from build123d import *

# Parameters (mm, degrees)
SKETCH1_R           = 3
BOSS_EXTRUDE1_DEPTH = 3
FILLET1_R           = 1.5
SKETCH2_R           = 1.5
BOSS_EXTRUDE2_DEPTH = 12.7


with BuildPart() as part:
    # Sketch1 → Boss-Extrude1 (new body)
    with BuildSketch(Plane(origin=(0, 0, 0), x_dir=(1, 0, 0), z_dir=(0, 1, 0))):
        Circle(SKETCH1_R)
    extrude(amount=BOSS_EXTRUDE1_DEPTH)

    # Fillet1
    fillet1_edges = [part.edges().sort_by_distance(p)[0] for p in [
        (-3, 3, 0),
    ]]
    fillet(fillet1_edges, radius=FILLET1_R)

    # Sketch2 → Boss-Extrude2 (add)
    with BuildSketch(Plane.XZ):
        Circle(SKETCH2_R)
    extrude(amount=BOSS_EXTRUDE2_DEPTH)


solid = part.part
Can you work these out from the model? Positions are in its coordinate system, mm. Give positions to 0.01 mm unless a question says otherwise; leave off trailing zeros. Write each loop counter-clockwise with the first axis right and the second up, starting at its lowest first coordinate (ties: lowest second). Pieces come first, ordered by that corner, then holes. Notation, with made-up numbers: M -26.75,-27 L 26.25,-27 A20 cw 26.25,-10 Z; hole C -7,3.25 d1. An arc over 180 degrees is marked long. Answer in a Markdown table with one row per item. Add a question column.
Item 1: For pin 1 Ø2 at (y, z) = (-4, -0.5) entering from +X, with a flat end and sliding along its axis, tell me the tip position at first contact or that it passes through.
Item 2: We'd pull the mould along Y, two halves only. Please class faces 1 (the flat face through (0, 3, 0)), 2 (the cylindrical face through (-1.5, -6.26, 0.07)), 3 (the flat face through (1.3, 0, 1.3)): released by +Y, released by -Y, zero draft, split by the parting line, or undercut.
Item 3: Please list where these lines run through material, in increasing order: L1, parallel to Y at x = 2.25, z = 0.75; L2, parallel to Y at x = 0.25, z = -1.75; L3, parallel to Z at x = -0.5, y = -7.75.
Item 4: Imagine slicing it at A-A, the plane y = -2.75. Write out the boundary of the cut face in (x, z), plus the area to 3 significant figures.
Evaluation:
| question | item | result |
|---|---|---|
| 1 | pin 1 | stops at x = 1.5 |
| 2 | face 1 | released by +Y |
| 2 | face 2 | zero draft |
| 2 | face 3 | released by -Y |
| 3 | L1 | y = 0 to 2.72 |
| 3 | L2 | y = 0 to 2.98 |
| 3 | L3 | z = -1.41 to 1.41 |
| 4 | outline | C 0,0 d3 |
| 4 | area | 7.07 mm² |
